Part model, mm, in its own coordinate system. Face numbers are marked on the shaded views. A direction names the side the tool comes from. Round coordinates to 2 decimals unless told otherwise and drop trailing zeros. Write each loop counter-clockwise with the first axis right and the second up, starting at its lowest first coordinate (ties: lowest second). Pieces come first, ordered by that corner, then holes. Notation, with made-up numbers: M 67,-31 L 112,-31 A13 ccw 112,-22 Z; hole C -8.75,-11 d1. An arc over 180 degrees is marked long. Answer as a JSON object with one key per item and string values. Group by question number.
1. Which spindle directions (+Z, -Z, +X, -X, +Y, -Y) get a long thin tool onto all of the face, cutting with end or side? Do the marked faces 4 and 5. Say none if no direction does.
2. Band-saw the part on B-B, the plane z = 1.15. Write the cut outline in (x, y).
3. Two-plate mould, pull along X, no slides. Class the marked faces 1, 2 and 3: +X half, -X half, draft (parallel to the pull), parting line (faces both ways), or undercut.
4. Band-saw the part on C-C, the plane x = 9. Write the cut outline in (y, z), plus the area to 3 significant figures.
5. Band-saw the part on A-A, the plane y = 0.5. Write the cut outline in (x, z), plus the area to 3 significant figures.
6. Drop flat-ended pins along their axis: pin 1 (1 mm diameter, centred on x = -13, y = 4, fed in from +Z); pin 2 (1.5 mm diameter, centred on x = -7, z = 4.5, fed in from +Y); pin 3 (3 mm diameter, centred on x = 16, y = 1.7, fed in from +Z). Give the stop position or say it passes through.
7. Drill centre lines: line 1 (X direction, y = 3, z = 2.1); line 2 (Y direction, x = 16, z = 1.55); line 3 (Y direction, x = -13, z = 4.85). Where is each one in solid material? Low to high. Write a range as from..to.
8. Band-saw the part on D-D, the plane z = 5.3. Write the cut outline in (x, y).
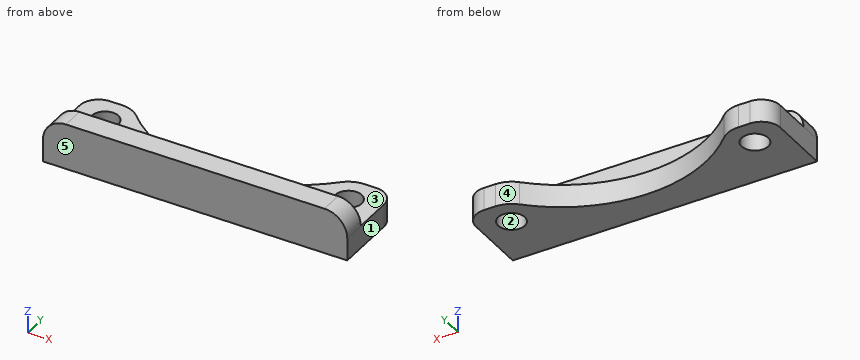
from build123d import *

# Parameters (mm, degrees)
ESBO_O1_W                = 40
ESBO_O1_H                = 10.6
RESSALTO_EXTRUS_O1_DEPTH = 3
ESBO_O2_W                = 40
ESBO_O2_H                = 3
RESSALTO_EXTRUS_O2_DEPTH = 3
FILETE1_R                = 3
ESBO_O3_R                = 1.75
CORTE_EXTRUS_O1_DEPTH    = 3
FILETE2_R                = 2.5
FILETE3_R                = 3.6


with BuildPart() as part:
    # Esboço1 → Ressalto-extrusão1 (new body)
    with BuildSketch(Plane.XY):
        Rectangle(ESBO_O1_W, ESBO_O1_H)
    extrude(amount=RESSALTO_EXTRUS_O1_DEPTH)

    # Esboço2 → Ressalto-extrusão2 (add)
    with BuildSketch(Plane.XY.offset(3)):
        with Locations((0, -3.8)):
            Rectangle(ESBO_O2_W, ESBO_O2_H)
    extrude(amount=RESSALTO_EXTRUS_O2_DEPTH)

    # Filete1
    filete1_edges = [part.edges().sort_by_distance(p)[0] for p in [
        (-20, -3.8, 6),
        (20, -3.8, 6),
    ]]
    fillet(filete1_edges, radius=FILETE1_R)

    # Esboço3 → Corte-extrusão1 (cut)
    with BuildSketch(Plane(origin=(0, 0, 0), x_dir=(-1, 0, 0), z_dir=(0, 0, -1))):
        with BuildLine():
            ThreePointArc((14.39583273, 5.3), (17.811805381, 11.086408762), (19, 17.7))
            ThreePointArc((19, 17.7), (-6.613591238, 35.511805381), (-14.39583273, 5.3))
            Line((-14.39583273, 5.3), (14.39583273, 5.3))
        make_face()
        with BuildLine():
            Line((14.39583273, 5.3), (-14.39583273, 5.3))
            ThreePointArc((-14.39583273, 5.3), (0, -1.3), (14.39583273, 5.3))
        make_face()
        with Locations((16, 1.7)):
            Circle(ESBO_O3_R)
        with Locations((-16, 1.7)):
            Circle(ESBO_O3_R)
    extrude(amount=-CORTE_EXTRUS_O1_DEPTH, mode=Mode.SUBTRACT)

    # Filete2
    filete2_edges = [part.edges().sort_by_distance(p)[0] for p in [
        (-20, 5.3, 1.5),
        (20, 5.3, 1.5),
    ]]
    fillet(filete2_edges, radius=FILETE2_R)

    # Filete3
    filete3_edges = [part.edges().sort_by_distance(p)[0] for p in [
        (-14.39583273, 5.3, 1.5),
        (14.39583273, 5.3, 1.5),
    ]]
    fillet(filete3_edges, radius=FILETE3_R)


solid = part.part
Worked answers:
{
 "1": {"face 4": "+Z, -Z, +Y", "face 5": "+Z, -Z, +X, -X, -Y"},
 "2": {"outline": "M -20,-5.3 L 20,-5.3 L 20,2.8 A2.5 ccw 17.5,5.3 L 15.96,5.3 A3.6 ccw 13.42,4.25 A19 cw -13.42,4.25 A3.6 ccw -15.96,5.3 L -17.5,5.3 A2.5 ccw -20,2.8 Z; hole C -16,1.7 d3.5; hole C 16,1.7 d3.5"},
 "3": {"face 1": "+X half", "face 2": "undercut", "face 3": "draft"},
 "4": {"outline": "M -5.3,0 L 0.97,0 L 0.97,3 L -2.3,3 L -2.3,6 L -5.3,6 Z", "area": "27.8 mm^2"},
 "5": {"outline": "M -20,0 L -17.27,0 L -17.27,3 L -20,3 Z; M -14.73,0 L -8.07,0 L -8.07,3 L -14.73,3 Z; M 8.07,0 L 14.73,0 L 14.73,3 L 8.07,3 Z; M 17.27,0 L 20,0 L 20,3 L 17.27,3 Z", "area": "56.3 mm^2"},
 "6": {"pin 1": "stops at z = 3", "pin 2": "stops at y = -2.3", "pin 3": "passes through"},
 "7": {"line 1": "x = -19.99..-17.17, -14.83..-12.04, 12.04..14.83, 17.17..19.99", "line 2": "y = -5.3..-0.05, 3.45..5.3", "line 3": "y = -5.3..-2.3"},
 "8": {"outline": "M -18.93,-5.3 L 18.93,-5.3 L 18.93,-2.3 L -18.93,-2.3 Z"}
}
